Geometry check sheet. Reference: the model listing, model coordinates, mm. A direction names the side the tool comes from. Round coordinates to 2 decimals unless told otherwise and drop trailing zeros. Loops run counter-clockwise (first coordinate to the right, second up) from the corner with the lowest first, then second, coordinate; pieces in that order, holes last. Notation, with made-up numbers: (23.5, -37.5) -> (55.5, -37.5) arc R28 cw to (55.5, -16.5) -> close; hole circle Ø4 at (28, 42.25). An arc over 180 degrees is marked (long way). Use one line per item in the form item = value.
from build123d import *

# Parameters (mm, degrees)
SKETCH1_R           = 7
BOSS_EXTRUDE1_DEPTH = 10
SKETCH2_W           = 2
SKETCH2_H           = 1
BOSS_EXTRUDE2_DEPTH = 4
CUT_EXTRUDE2_DEPTH  = 10
FILLET1_R           = 1
FILLET2_R           = 0.5
CUT_EXTRUDE4_DEPTH  = 10
SKETCH5_W           = 3.959584723
SKETCH5_H           = 3
BOSS_EXTRUDE3_DEPTH = 7
FILLET3_R           = 0.5
FILLET4_R           = 0.5


# Some blends are built 0.0001 mm under size
with BuildPart() as part:
    # Sketch1 → Boss-Extrude1 (new body)
    with BuildSketch(Plane(origin=(0, 0, 0), x_dir=(1, 0, 0), z_dir=(0, 1, 0))):
        with Locations(Location((0, 0, 0), (0, 0, 270))):
            Circle(SKETCH1_R)
    extrude(amount=BOSS_EXTRUDE1_DEPTH)

    # Sketch2 → Boss-Extrude2 (add)
    with BuildSketch(Plane(origin=(0, 10, 0), x_dir=(1, 0, 0), z_dir=(0, 1, 0))):
        with Locations((-1, 1.5)):
            Rectangle(SKETCH2_W, SKETCH2_H)
        with Locations((1, 1.5)):
            Rectangle(SKETCH2_W, SKETCH2_H)
        with Locations((1, -1.5)):
            Rectangle(SKETCH2_W, SKETCH2_H)
        with Locations((-1, -1.5)):
            Rectangle(SKETCH2_W, SKETCH2_H)
    extrude(amount=BOSS_EXTRUDE2_DEPTH)

    # Sketch3 → Cut-Extrude2 (cut)
    with BuildSketch(Plane.XY.offset(2)):
        with BuildLine():
            Line((2, 14), (0, 14))
            ThreePointArc((0, 14), (1.414213562, 13.414213562), (2, 12))
            Line((2, 12), (2, 14))
        make_face()
        with BuildLine():
            Line((0, 14), (-2, 14))
            Line((-2, 14), (-1.414213562, 13.414213562))
            ThreePointArc((-1.414213562, 13.414213562), (-0.765366865, 13.847759065), (0, 14))
        make_face()
        with BuildLine():
            Line((-1.414213562, 13.414213562), (-2, 14))
            Line((-2, 14), (-2, 12))
            ThreePointArc((-2, 12), (-1.847759065, 12.765366865), (-1.414213562, 13.414213562))
        make_face()
        with BuildLine():
            ThreePointArc((0.75, 12), (0.287012574, 12.692909649), (-0.530330086, 12.530330086))
            Line((-0.530330086, 12.530330086), (0.530330086, 11.469669914))
            ThreePointArc((0.530330086, 11.469669914), (0.692909649, 11.712987426), (0.75, 12))
        make_face()
        with BuildLine():
            Line((0.530330086, 11.469669914), (-0.530330086, 12.530330086))
            ThreePointArc((-0.530330086, 12.530330086), (-0.530330086, 11.469669914), (0.530330086, 11.469669914))
        make_face()
    extrude(amount=-CUT_EXTRUDE2_DEPTH, mode=Mode.SUBTRACT)

    # Fillet1
    fillet1_edges = [part.edges().sort_by_distance(p)[0] for p in [
        (0, 10, -7),
    ]]
    fillet(fillet1_edges, radius=FILLET1_R)

    # Fillet2
    fillet2_edges = [part.edges().sort_by_distance(p)[0] for p in [
        (2, 11, 1),
        (-2, 11, 1),
        (2, 11, 2),
        (-2, 11, 2),
        (-2, 11, -2),
        (2, 11, -2),
        (-2, 11, -1),
        (2, 11, -1),
        (0, 14, 1),
        (0, 14, 2),
        (0, 14, -2),
        (0, 14, -1),
    ]]
    fillet(fillet2_edges, radius=FILLET2_R - 0.0001)  # a hair under: the kernel refuses the full size

    # Sketch4 → Cut-Extrude4 (cut, symmetric)
    with BuildSketch(Plane.XY):
        Polygon((-7, 4), (7, 4), (9.323554176, 4), (9.323554176, 10.076967931), (-7.870406088, 10.076967931), (-7.870406088, 4), align=None)
    extrude(amount=CUT_EXTRUDE4_DEPTH, both=True, mode=Mode.SUBTRACT)


with BuildPart() as cut_extrude4_piece_1:
    # of the separate pieces the step leaves, piece 1, a body of its own (cut_extrude4_pieces)
    add(part.part.solids().sort_by_distance((0, 0, 7))[0])



with BuildPart() as cut_extrude4_piece_2:
    # of the separate pieces the step leaves, piece 2, a body of its own (cut_extrude4_pieces)
    add(part.part.solids().sort_by_distance((-1.5001, 10.076967931, 2))[0])


with BuildPart() as cut_extrude4_piece_3:
    # of the separate pieces the step leaves, piece 3, a body of its own (cut_extrude4_pieces)
    add(part.part.solids().sort_by_distance((-2, 10.076967931, -1.5001))[0])


with BuildPart() as cut_extrude4_piece_1_1:
    add(cut_extrude4_piece_1.part)

    add(cut_extrude4_piece_2.part)  # Boss-Extrude3 merges Cut-Extrude4 piece 2

    add(cut_extrude4_piece_3.part)  # Boss-Extrude3 merges Cut-Extrude4 piece 3
    # Sketch5 → Boss-Extrude3 (add)
    with BuildSketch(Plane(origin=(0, 4, 0), x_dir=(1, 0, 0), z_dir=(0, 1, 0))):
        with Locations((0.009752672, 0)):
            Rectangle(SKETCH5_W, SKETCH5_H)
    extrude(amount=BOSS_EXTRUDE3_DEPTH)

    # Fillet3
    fillet3_edges = [cut_extrude4_piece_1_1.edges().sort_by_distance(p)[0] for p in [
        (-1.97003969, 11, 0),
        (1.989545033, 11, 0),
    ]]
    fillet(fillet3_edges, radius=FILLET3_R)

    # Fillet4
    # the kernel refuses this fillet: 0.5 mm, written as the material it takes off along each edge
    with BuildSketch(Plane(origin=(-1.97003969, 4, 1.5), x_dir=(0, 0, -1), z_dir=(0, 1, 0)), Plane(origin=(1.989545033, 4, 1.5), x_dir=(-1, 0, 0), z_dir=(0, 1, 0))) as fillet4_piece_1:
        with BuildLine():
            CenterArc((FILLET4_R, -FILLET4_R), FILLET4_R, 90, 90)
            Line((0, -FILLET4_R), (0, 0))
            Line((0, 0), (FILLET4_R, 0))
        make_face()
    extrude(amount=6.076967931, mode=Mode.SUBTRACT)
    with BuildSketch(Plane(origin=(-1.97003969, 4, 1.5), x_dir=(0, 0, -1), z_dir=(0, 1, 0))) as fillet4_piece_2_section:
        with BuildLine():
            CenterArc((FILLET4_R, -FILLET4_R), FILLET4_R, 90, 90)
            Line((0, -FILLET4_R), (0, 0))
            Line((0, 0), (FILLET4_R, 0))
        make_face()
    fillet4_piece_2 = extrude(amount=7.326967931, mode=Mode.PRIVATE)
    fillet4_piece_2 = fillet4_piece_2 - Plane(origin=(-1.47003969, 10.5, 1.201598319), x_dir=(-1, 0, 0), z_dir=(0, 0, -1)) * Cylinder(0.5, 17, mode=Mode.PRIVATE)
    fillet4_piece_2 = fillet4_piece_2 - Plane(origin=(-1.5001, 10.234965589, 1.4999), x_dir=(-1, 0, 0), z_dir=(0, -1, 0)) * Cylinder(0.4999, 17, mode=Mode.PRIVATE)
    add(fillet4_piece_2, mode=Mode.SUBTRACT)
    with BuildSketch(Plane(origin=(-1.97003969, 4, -1.5), x_dir=(0, 0, 1), z_dir=(0, 1, 0)), Plane(origin=(1.989545033, 4, -1.5), x_dir=(-1, 0, 0), z_dir=(0, 1, 0))) as fillet4_piece_3:
        with BuildLine():
            CenterArc((FILLET4_R, FILLET4_R), FILLET4_R, 180, 90)
            Line((0, FILLET4_R), (0, 0))
            Line((0, 0), (FILLET4_R, 0))
        make_face()
    extrude(amount=6.076967931, mode=Mode.SUBTRACT)
    with BuildSketch(Plane(origin=(-1.97003969, 4, -1.5), x_dir=(0, 0, 1), z_dir=(0, 1, 0))) as fillet4_piece_4_section:
        with BuildLine():
            CenterArc((FILLET4_R, FILLET4_R), FILLET4_R, 180, 90)
            Line((0, FILLET4_R), (0, 0))
            Line((0, 0), (FILLET4_R, 0))
        make_face()
    fillet4_piece_4 = extrude(amount=7.326967931, mode=Mode.PRIVATE)
    fillet4_piece_4 = fillet4_piece_4 - Plane(origin=(-1.5001, 10.234965589, -1.4999), x_dir=(-1, 0, 0), z_dir=(0, 1, 0)) * Cylinder(0.4999, 17, mode=Mode.PRIVATE)
    fillet4_piece_4 = fillet4_piece_4 - Plane(origin=(-1.47003969, 10.5, -1.201598319), x_dir=(-1, 0, 0), z_dir=(0, 0, -1)) * Cylinder(0.5, 17, mode=Mode.PRIVATE)
    add(fillet4_piece_4, mode=Mode.SUBTRACT)
    with BuildSketch(Plane(origin=(1.989545033, 4, -1.5), x_dir=(-1, 0, 0), z_dir=(0, 1, 0))) as fillet4_piece_5_section:
        with BuildLine():
            CenterArc((FILLET4_R, FILLET4_R), FILLET4_R, 180, 90)
            Line((0, FILLET4_R), (0, 0))
            Line((0, 0), (FILLET4_R, 0))
        make_face()
    fillet4_piece_5 = extrude(amount=7.326967931, mode=Mode.PRIVATE)
    fillet4_piece_5 = fillet4_piece_5 - Plane(origin=(1.489545033, 10.5, -1.228788283), x_dir=(1, 0, 0), z_dir=(0, 0, 1)) * Cylinder(0.5, 17, mode=Mode.PRIVATE)
    fillet4_piece_5 = fillet4_piece_5 - Plane(origin=(1.5001, 10.231594364, -1.4999), x_dir=(1, 0, 0), z_dir=(0, -1, 0)) * Cylinder(0.4999, 17, mode=Mode.PRIVATE)
    add(fillet4_piece_5, mode=Mode.SUBTRACT)
    with BuildSketch(Plane(origin=(1.989545033, 4, 1.5), x_dir=(-1, 0, 0), z_dir=(0, 1, 0))) as fillet4_piece_6_section:
        with BuildLine():
            CenterArc((FILLET4_R, -FILLET4_R), FILLET4_R, 90, 90)
            Line((0, -FILLET4_R), (0, 0))
            Line((0, 0), (FILLET4_R, 0))
        make_face()
    fillet4_piece_6 = extrude(amount=7.326967931, mode=Mode.PRIVATE)
    fillet4_piece_6 = fillet4_piece_6 - Plane(origin=(1.489545033, 10.5, 1.228788283), x_dir=(1, 0, 0), z_dir=(0, 0, 1)) * Cylinder(0.5, 17, mode=Mode.PRIVATE)
    fillet4_piece_6 = fillet4_piece_6 - Plane(origin=(1.5001, 10.231594364, 1.4999), x_dir=(1, 0, 0), z_dir=(0, 1, 0)) * Cylinder(0.4999, 17, mode=Mode.PRIVATE)
    add(fillet4_piece_6, mode=Mode.SUBTRACT)
    # the kernel refuses this fillet: 0.5 mm, written as the material it adds along each edge
    with BuildSketch(Plane(origin=(-1.97003969, 4, 1), x_dir=(0, 1, 0), z_dir=(0, 0, -1)), Plane(origin=(1.989545033, 4, -1), x_dir=(0, 1, 0), z_dir=(0, 0, 1))) as fillet4_2_piece_1:
        with BuildLine():
            CenterArc((FILLET4_R, -FILLET4_R), FILLET4_R, 90, 90)
            Line((0, -FILLET4_R), (0, 0))
            Line((0, 0), (FILLET4_R, 0))
        make_face()
    extrude(amount=2)
    with BuildSketch(Plane(origin=(-1.47003969, 4, -1.5), x_dir=(0, 0, -1), z_dir=(1, 0, 0))) as fillet4_2_piece_2:
        with BuildLine():
            CenterArc((FILLET4_R, FILLET4_R), FILLET4_R, 180, 90)
            Line((0, FILLET4_R), (0, 0))
            Line((0, 0), (FILLET4_R, 0))
        make_face()
    extrude(amount=2.959584723)
    with BuildSketch(Plane(origin=(1.489545033, 4, 1.5), x_dir=(0, 1, 0), z_dir=(-1, 0, 0))) as fillet4_2_piece_3:
        with BuildLine():
            CenterArc((FILLET4_R, -FILLET4_R), FILLET4_R, 90, 90)
            Line((0, -FILLET4_R), (0, 0))
            Line((0, 0), (FILLET4_R, 0))
        make_face()
    extrude(amount=2.959584723)
    with BuildSketch(Plane(origin=(1.489545033, 4, -1), x_dir=(0, 0, -1), z_dir=(-1, 0, 0))) as fillet4_2_piece_4:
        with BuildLine():
            CenterArc((0.5 + FILLET4_R, -FILLET4_R), FILLET4_R, 90, 90)
            Line((0.5 + FILLET4_R, 0), (0.5, 0))
            Line((0.5, 0), (0.5, -FILLET4_R))
        make_face()
    revolve(axis=Axis((1.489545033, 4, -1), (0, -1, 0)), revolution_arc=90)
    with BuildSketch(Plane(origin=(1.489545033, 4, 1), x_dir=(1, 0, 0), z_dir=(0, 0, -1))) as fillet4_2_piece_5:
        with BuildLine():
            CenterArc((0.5 + FILLET4_R, -FILLET4_R), FILLET4_R, 90, 90)
            Line((0.5 + FILLET4_R, 0), (0.5, 0))
            Line((0.5, 0), (0.5, -FILLET4_R))
        make_face()
    revolve(axis=Axis((1.489545033, 4, 1), (0, -1, 0)), revolution_arc=90)
    with BuildSketch(Plane(origin=(-1.47003969, 4, 1), x_dir=(-1, 0, 0), z_dir=(0, 0, -1))) as fillet4_2_piece_6:
        with BuildLine():
            CenterArc((0.5 + FILLET4_R, FILLET4_R), FILLET4_R, 180, 90)
            Line((0.5 + FILLET4_R, 0), (0.5, 0))
            Line((0.5, 0), (0.5, FILLET4_R))
        make_face()
    revolve(axis=Axis((-1.47003969, 4, 1), (0, 1, 0)), revolution_arc=90)
    with BuildSketch(Plane(origin=(-1.47003969, 4, -1), x_dir=(0, 0, -1), z_dir=(1, 0, 0))) as fillet4_2_piece_7:
        with BuildLine():
            CenterArc((0.5 + FILLET4_R, FILLET4_R), FILLET4_R, 180, 90)
            Line((0.5 + FILLET4_R, 0), (0.5, 0))
            Line((0.5, 0), (0.5, FILLET4_R))
        make_face()
    revolve(axis=Axis((-1.47003969, 4, -1), (0, 1, 0)), revolution_arc=90)


solid = cut_extrude4_piece_1_1.part
1. Material ranges on line 1 along Z through (x, y) = (-0.75, 13.25); line 2 along Y through (x, z) = (-5.25, 0); line 3 along Z through (x, y) = (0.75, 2), recorded low to high.
Return value:
line_1 = -2 to -1, 1 to 2
line_2 = 0 to 4
line_3 = -6.96 to 6.96
2. Gauge pin test, flat ends, axial feed: pin 1 (0.9 mm diameter, centred on x = -0.5, y = 6.5, fed in from +Z); pin 2 (1.6 mm diameter, centred on x = -0.5, z = 0, fed in from +Y); pin 3 (2 mm diameter, centred on y = 8.5, z = 0, fed in from -X). Record the tip position at first contact, or that the pin passes through.
Return value:
pin_1 = 1.5
pin_2 = 11
pin_3 = -1.97
3. Section check B-B (z = 0). Record the boundary of the cut face in (x, y), then the cut area to 3 significant figures.
Return value:
outline = (-7, 0) -> (7, 0) -> (7, 4) -> (2.49, 4) arc R0.5 cw to (1.99, 4.5) -> (1.99, 10.5) arc R0.5 ccw to (1.49, 11) -> (-1.47, 11) arc R0.5 ccw to (-1.97, 10.5) -> (-1.97, 4.5) arc R0.5 cw to (-2.47, 4) -> (-7, 4) -> close
area = 83.7 mm2
4. Tool access check on faces 1 (the flat face through (0, 0, 0)), 2 (the flat face through (0, 7, 1.5)), 3 (the flat face through (3, 4, 0)), 4 (the flat face through (0, 11, -2)), 5 (the flat face through (0, 11, 0)). Record the directions out of +Z, -Z, +X, -X, +Y, -Y that give a thin tool (end or side, any length) a straight path to the whole face; none if there is none.
Return value:
face_1 = +Z, -Z, +X, -X, -Y
face_2 = +Z, +X, -X
face_3 = +Y
face_4 = -Z, +X, -X, +Y
face_5 = +X, -X, +Y
5. Section check A-A (y = 8.75). Record the boundary of the cut face in (x, z).
Return value:
outline = (-1.97, -1) arc R0.5 ccw to (-1.47, -1.5) -> (1.49, -1.5) arc R0.5 ccw to (1.99, -1) -> (1.99, 1) arc R0.5 ccw to (1.49, 1.5) -> (-1.47, 1.5) arc R0.5 ccw to (-1.97, 1) -> close
6. Section check D-D (y = 2.25). Record the boundary of the cut face in (x, z).
Return value:
outline = circle Ø14 at (0, 0)
7. Section check C-C (x = -5.25). Record the boundary of the cut face in (y, z), then the cut area to 3 significant figures.
Return value:
outline = (0, -4.63) -> (4, -4.63) -> (4, 4.63) -> (0, 4.63) -> close
area = 37.0 mm2
8. Mould release check, pull along Z, two halves, no side actions. Record for faces 6 (the flat face through (0, 13, -1)), 7 (the flat face through (0, 13, 1)), 8 (the flat face through (0, 7, -1.5)), 9 (the flat face through (0, 11, 2)): released by +Z, released by -Z, zero draft, split by the parting line, or undercut.
Return value:
face_6 = undercut
face_7 = undercut
face_8 = released by -Z
face_9 = released by +Z
